Source: three-view drawing plus pictorial views. Frame: mm from the lowest corner of the part. Give positions to 0.01 mm unless a question says otherwise; leave off trailing zeros. Loops run counter-clockwise (first coordinate to the right, second up) from the corner with the lowest first, then second, coordinate; pieces in that order, holes last. Notation, with made-up numbers: (-37.5, 59) - (12.5, 59) arc R15 ccw to (12.5, 75) - close; hole circle Ø5 at (81.5, 63.5). An arc over 180 degrees is marked (long way). Answer as a JSON object with one key per item and string values.
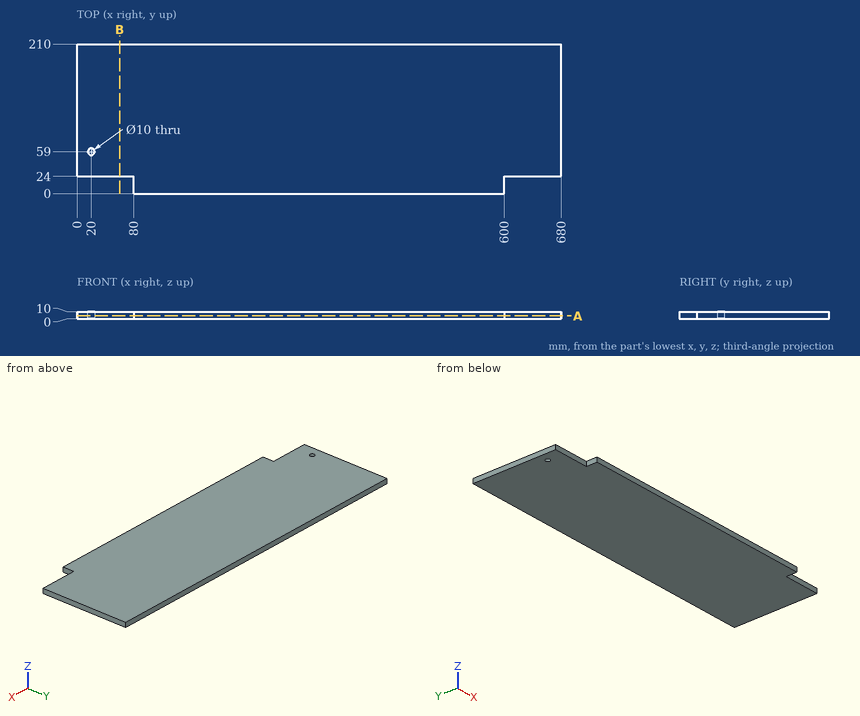
Item 1: Cut plane B-B (x = 60). Return loops of the section in (y, z).
Geometry check:
{"outline": "(24, 0) - (210, 0) - (210, 10) - (24, 10) - close"}
Item 2: Cut plane A-A (z = 4). Return loops of the section in (x, y), then the cut area to 3 significant figures.
Geometry check:
{"outline": "(0, 24) - (80, 24) - (80, 0) - (600, 0) - (600, 24) - (680, 24) - (680, 210) - (0, 210) - close; hole circle Ø10 at (20, 59)", "area": "139,000 mm2"}
Item 3: Contact query for flat-ended pins moving along their axis: P1, Ø5, axis at y = 15.5, z = 3.5, coming from the +X side; P2, Ø5, axis at x = 648.5, z = 3, coming from the -Y side; P3, Ø4, axis at x = 574, y = 121, coming from the -Z side. Output: stop coordinate, or through.
Geometry check:
{"P1": "stops at x = 600", "P2": "stops at y = 24", "P3": "stops at z = 0"}
Item 4: Material intervals for line 1 (X direction, y = 16.5, z = 2); line 2 (Y direction, x = 20, z = 6.25); line 3 (Y direction, x = 28, z = 6.75), sorted ascending. Write a range as [from, to].
Geometry check:
{"line 1": "x = [80, 600]", "line 2": "y = [24, 54], [64, 210]", "line 3": "y = [24, 210]"}
